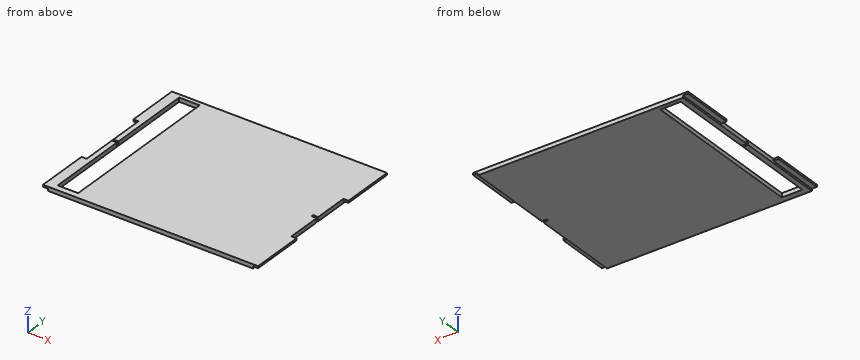
from build123d import *

# Parameters (mm, degrees)
EXTRUDE_1_DEPTH          = 2
SKETCH_2_W               = 200
SKETCH_2_H               = 174
SKETCH_2_W_2             = 20
SKETCH_2_H_2             = 164
EXTRUDE_2_DEPTH          = 2
CUT_EXTRUDE_1_DEPTH      = 137.759825972
CUT_EXTRUDE_1_DEPTH_BACK = 137.759825972
SKETCH_3_W               = 5
SKETCH_3_H               = 2


with BuildPart() as part:
    # 草图1 → 凸台-拉伸1 (new body)
    with BuildSketch(Plane.XY):
        Polygon((104.5, 35), (104.5, 87), (-105.5, 87), (-105.5, 35), (-100.5, 35), (-100.5, -35), (-105.5, -35), (-105.5, -87), (104.5, -87), (104.5, -35), (99.5, -35), (99.5, 35), align=None)
        Polygon((-95.5, 35), (-95.5, 83), (-75.5, 83), (-75.5, -81), (-95.5, -81), align=None, mode=Mode.SUBTRACT)
    extrude(amount=EXTRUDE_1_DEPTH)

    # 草图2 → 凸台-拉伸2 (add)
    with BuildSketch(Plane.XY):
        with Locations((-0.5, 0)):
            Rectangle(SKETCH_2_W, SKETCH_2_H)
        with Locations((-85.5, 1)):
            Rectangle(SKETCH_2_W_2, SKETCH_2_H_2, mode=Mode.SUBTRACT)
    extrude(amount=-EXTRUDE_2_DEPTH)

    # 草图3 → 切除-拉伸1 (cut, two sides: drawn at the far end of the back side and taken through both)
    with BuildSketch(Plane.XY.offset(-CUT_EXTRUDE_1_DEPTH_BACK)):
        with Locations((-98, 0)):
            Rectangle(SKETCH_3_W, SKETCH_3_H)
        Polygon((99.5, 0), (99.5, 1), (94.5, 1), (94.5, -1), (99.5, -1), align=None)
    extrude(amount=CUT_EXTRUDE_1_DEPTH + CUT_EXTRUDE_1_DEPTH_BACK, mode=Mode.SUBTRACT)


solid = part.part
Verification items for the finished model (mm, model axes). Coordinates: 2 decimals unless noted, no trailing zeros. Write each loop counter-clockwise with the first axis right and the second up, starting at its lowest first coordinate (ties: lowest second). Pieces come first, ordered by that corner, then holes. Notation, with made-up numbers: M -36.75,67 L 20.25,67 A34 cw 20.25,98 Z; hole C 30,-22.75 d5. An arc over 180 degrees is marked long. Use CSV: the item, a comma, the result in double quotes.
Q1. Section check D-D, the plane y = -5. Enter the section's corners in (x, z).
Computed values:
outline,"M -100.5,-2 L -95.5,-2 L -95.5,2 L -100.5,2 Z; M -75.5,-2 L 99.5,-2 L 99.5,2 L -75.5,2 Z"
Q2. Section check A-A, the plane y = 65.5. Enter the section's corners in (x, z).
Computed values:
outline,"M -105.5,0 L -100.5,0 L -100.5,-2 L -95.5,-2 L -95.5,2 L -105.5,2 Z; M -75.5,-2 L 99.5,-2 L 99.5,0 L 104.5,0 L 104.5,2 L -75.5,2 Z"
Q3. Section check C-C, the plane z = 0.75. Enter the section's corners in (x, y).
Computed values:
outline,"M -105.5,-87 L 104.5,-87 L 104.5,-35 L 99.5,-35 L 99.5,-1 L 94.5,-1 L 94.5,1 L 99.5,1 L 99.5,35 L 104.5,35 L 104.5,87 L -105.5,87 L -105.5,35 L -100.5,35 L -100.5,1 L -95.5,1 L -95.5,83 L -75.5,83 L -75.5,-81 L -95.5,-81 L -95.5,-1 L -100.5,-1 L -100.5,-35 L -105.5,-35 Z"
Q4. Section check B-B, the plane x = -79. Enter the section's corners in (y, z).
Computed values:
outline,"M -87,-2 L -81,-2 L -81,2 L -87,2 Z; M 83,-2 L 87,-2 L 87,2 L 83,2 Z"
Q5. Thickness scan on line 1 along Y through (x, z) = (-79.5, -0.5); line 2 along X through (y, z) = (19, -1.3); line 3 along X through (y, z) = (-59, 0.4). Record the ranges inside material, lowest first. Write a range as [from, to].
Computed values:
line 1,"[-87, -81], [83, 87]"
line 2,"[-100.5, -95.5], [-75.5, 99.5]"
line 3,"[-105.5, -95.5], [-75.5, 104.5]"
Q6. Go/stop test with flat-tipped pins: P1, Ø1.6, axis at y = 0, z = 0.5, coming from the +X side; P2, Ø2.5, axis at x = -103, y = -70.5, coming from the -Z side; P3, Ø1.5, axis at y = -45, z = -1, coming from the +X side. Record where each tip stops, or that it passes through.
Computed values:
P1,"x = 94.5"
P2,"z = 0"
P3,"x = 99.5"
